The listing builds one solid part. Answer for the finished solid, in the listing's coordinates (mm). A direction names the side the tool comes from. Round coordinates to 2 decimals unless told otherwise and drop trailing zeros. Loops run counter-clockwise (first coordinate to the right, second up) from the corner with the lowest first, then second, coordinate; pieces in that order, holes last. Notation, with made-up numbers: (-6.5, 71.25) -> (0.5, 71.25) arc R27 cw to (0.5, 93.25) -> close; hole circle Ø6 at (82, -9). An arc over 180 degrees is marked (long way). Use a Markdown table: item, result. Add a question column.
Q1. Section D-D on y = -21.5 is taken. Give the vertices of the cut face in (x, z), then the cut area to 3 significant figures.
Q2. Section C-C on z = 58 is taken. Give the vertices of the cut face in (x, y), then the cut area to 3 significant figures.
Q3. Section A-A on z = 21 is taken. Give the vertices of the cut face in (x, y), then the cut area to 3 significant figures.
Q4. Consider line 1 (X direction, y = 0, z = 58); line 2 (Y direction, x = 0, z = 51); line 3 (X direction, y = -2.5, z = 30). Determine where each line is inside the solid, lowest interval first.
Q5. Given pin 1 Ø2 at (y, z) = (16.5, 54) entering from -X; pin 2 Ø1 at (x, z) = (-12.5, 43.5) entering from +Y; pin 3 Ø5 at (y, z) = (17.5, 57) entering from -X, each flat-ended and moving along its own axis, determine where each tip first touches the part or whether it passes through.
Q6. For a pull along X with two mould halves and no side action, classify faces 3 (the conical face through (-12.24, -5.08, 43.75)), 4 (the flat face through (11.661, 19.826, 32.538)), 5 (the flat face through (-23, 0, 33)) as released by +X, released by -X, zero draft, split by the parting line, or undercut.
Q7. Section B-B on y = 0 is taken. Give the vertices of the cut face in (x, z).
Q8. Which of the six approach directions +Z, -Z, +X, -X, +Y, -Y give full straight-line access (tool end or side, diameter ignored) to faces 1 (the cylindrical face through (14.985, 0.66, 19.72)), 2 (the flat face through (-11.34, 20.01, 32.54))?
from build123d import *

# Parameters (mm, degrees)
EXTRUDE_1_DEPTH     = 66
SKETCH_12_R         = 15
CUT_EXTRUDE_3_DEPTH = 40
SKETCH_16_R         = 15
CUT_EXTRUDE_6_DEPTH = 4
CUT_EXTRUDE_6_DRAFT = -25
SKETCH_17_R         = 13.134769367
CUT_EXTRUDE_7_DEPTH = 2
CUT_EXTRUDE_7_DRAFT = -40
SKETCH_18_R         = 12
CUT_EXTRUDE_8_DEPTH = 22


with BuildPart() as part:
    # 草图2 → 拉伸1 (new body)
    with BuildSketch(Plane.XY):
        Polygon((0, 26.558112383), (-23, 13.279056191), (-23, -13.279056191), (0, -26.558112383), (23, -13.279056191), (23, 13.279056191), align=None)
    extrude(amount=EXTRUDE_1_DEPTH)

    # 草图12 → 拉伸3 (cut)
    with BuildSketch(Plane(origin=(0, 0, 0), x_dir=(-1, 0, 0), z_dir=(0, 0, -1))):
        Circle(SKETCH_12_R)
    extrude(amount=-CUT_EXTRUDE_3_DEPTH, mode=Mode.SUBTRACT)


with BuildPart() as cut_extrude_6_tool:
    # 草图16 → 拉伸6 (with draft: the straight prism first)
    with BuildSketch(Plane(origin=(0, 0, 40), x_dir=(-1, 0, 0), z_dir=(0, 0, -1))):
        Circle(SKETCH_16_R)
    extrude(amount=-CUT_EXTRUDE_6_DEPTH)
    # 拉伸6: the draft: its side faces are tilted about the plane it starts from
    cut_extrude_6_sides = [cut_extrude_6_tool.faces().sort_by_distance(p)[0] for p in [
        (15, 0, 42),
    ]]
    draft(cut_extrude_6_sides, Plane(origin=(0, 0, 40), x_dir=(-1, 0, 0), z_dir=(0, 0, -1)), CUT_EXTRUDE_6_DRAFT)


with BuildPart() as part_1:
    add(part.part)

    # 拉伸6: cut by cut_extrude_6_tool
    add(cut_extrude_6_tool.part, mode=Mode.SUBTRACT)


with BuildPart() as cut_extrude_7_tool:
    # 草图17 → 拉伸7 (with draft: the straight prism first)
    with BuildSketch(Plane(origin=(0, 0, 44), x_dir=(-1, 0, 0), z_dir=(0, 0, -1))):
        Circle(SKETCH_17_R)
    extrude(amount=-CUT_EXTRUDE_7_DEPTH)
    # 拉伸7: the draft: its side faces are tilted about the plane it starts from
    cut_extrude_7_sides = [cut_extrude_7_tool.faces().sort_by_distance(p)[0] for p in [
        (13.134769367, 0, 45),
    ]]
    draft(cut_extrude_7_sides, Plane(origin=(0, 0, 44), x_dir=(-1, 0, 0), z_dir=(0, 0, -1)), CUT_EXTRUDE_7_DRAFT)


with BuildPart() as part_2:
    add(part_1.part)

    # 拉伸7: cut by cut_extrude_7_tool
    add(cut_extrude_7_tool.part, mode=Mode.SUBTRACT)

    # 草图18 → 拉伸8 (cut)
    with BuildSketch(Plane.XY.offset(66)):
        Circle(SKETCH_18_R)
    extrude(amount=-CUT_EXTRUDE_8_DEPTH, mode=Mode.SUBTRACT)


solid = part_2.part
Checked values:
| question | item | result |
|---|---|---|
| 1 | outline | (-8.76, 0) -> (8.76, 0) -> (8.76, 66) -> (-8.76, 66) -> close |
| 1 | area | 1,160 mm2 |
| 2 | outline | (-23, -13.28) -> (0, -26.56) -> (23, -13.28) -> (23, 13.28) -> (0, 26.56) -> (-23, 13.28) -> close; hole circle Ø24 at (0, 0) |
| 2 | area | 1,380 mm2 |
| 3 | outline | (-23, -13.28) -> (0, -26.56) -> (23, -13.28) -> (23, 13.28) -> (0, 26.56) -> (-23, 13.28) -> close; hole circle Ø30 at (0, 0) |
| 3 | area | 1,130 mm2 |
| 4 | line 1 | x = -23 to -12, 12 to 23 |
| 4 | line 2 | y = -26.56 to -12, 12 to 26.56 |
| 4 | line 3 | x = -23 to -14.79, 14.79 to 23 |
| 5 | pin 1 | stops at x = -19.15 |
| 5 | pin 2 | stops at y = 19.63 |
| 5 | pin 3 | stops at x = -20.02 |
| 6 | face 3 | undercut |
| 6 | face 4 | released by +X |
| 6 | face 5 | released by -X |
| 7 | outline | (-23, 0) -> (-15, 0) -> (-15, 40) -> (-13.13, 44) -> (-12, 45.35) -> (-12, 66) -> (-23, 66) -> close; (12, 45.35) -> (13.13, 44) -> (15, 40) -> (15, 0) -> (23, 0) -> (23, 66) -> (12, 66) -> close |
| 8 | face 1 | -Z |
| 8 | face 2 | +Z, -Z, -X, +Y |
